from build123d import *

# Parameters (mm, degrees)
ESQUISSE1_W             = 230
ESQUISSE1_H             = 350
BASE_EXTRUSION_DEPTH    = 1.5
ESQUISSE2_R             = 2.5
ENL_V_MAT_EXTRU_1_DEPTH = 1.5
ESQUISSE3_R             = 11.25
ENL_V_MAT_EXTRU_2_DEPTH = 1.5
ESQUISSE4_R             = 6.25
ENL_V_MAT_EXTRU_3_DEPTH = 1.5
ESQUISSE5_W             = 106
ESQUISSE5_H             = 131
ENL_V_MAT_EXTRU_4_DEPTH = 1.5
ESQUISSE6_W             = 37
ESQUISSE6_H             = 46
ENL_V_MAT_EXTRU_5_DEPTH = 1.5


with BuildPart() as part:
    # Esquisse1 → Base-Extrusion (new body)
    with BuildSketch(Plane.XY):
        with Locations((115, 175)):
            Rectangle(ESQUISSE1_W, ESQUISSE1_H)
    extrude(amount=BASE_EXTRUSION_DEPTH)

    # Esquisse2 → Enlèv. mat.-Extru.1 (cut)
    with BuildSketch(Plane.XY.offset(1.5)):
        with Locations((7, 7)):
            Circle(ESQUISSE2_R)
        with Locations((223, 7)):
            Circle(ESQUISSE2_R)
        with Locations((7, 343)):
            Circle(ESQUISSE2_R)
        with Locations((223, 343)):
            Circle(ESQUISSE2_R)
    extrude(amount=-ENL_V_MAT_EXTRU_1_DEPTH, mode=Mode.SUBTRACT)

    # Esquisse3 → Enlèv. mat.-Extru.2 (cut)
    with BuildSketch(Plane.XY.offset(1.5)):
        with Locations((45, 65)):
            Circle(ESQUISSE3_R)
        with Locations((45, 115)):
            Circle(ESQUISSE3_R)
        with Locations((45, 165)):
            Circle(ESQUISSE3_R)
        with Locations((45, 305)):
            Circle(ESQUISSE3_R)
        with BuildLine():
            Line((43.5, 251.14955156), (43.5, 253))
            Line((43.5, 253), (46.5, 253))
            Line((46.5, 253), (46.5, 251.14955156))
            ThreePointArc((46.5, 251.14955156), (45, 228.75), (43.5, 251.14955156))
        make_face()
    extrude(amount=-ENL_V_MAT_EXTRU_2_DEPTH, mode=Mode.SUBTRACT)

    # Esquisse4 → Enlèv. mat.-Extru.3 (cut)
    with BuildSketch(Plane.XY.offset(1.5)):
        with Locations((130, 70)):
            Circle(ESQUISSE4_R)
        with Locations((130, 89)):
            Circle(ESQUISSE4_R)
        with Locations((160, 70)):
            Circle(ESQUISSE4_R)
        with Locations((160, 89)):
            Circle(ESQUISSE4_R)
        with Locations((190, 70)):
            Circle(ESQUISSE4_R)
        with Locations((190, 89)):
            Circle(ESQUISSE4_R)
    extrude(amount=-ENL_V_MAT_EXTRU_3_DEPTH, mode=Mode.SUBTRACT)

    # Esquisse5 → Enlèv. mat.-Extru.4 (cut)
    with BuildSketch(Plane.XY.offset(1.5)):
        with Locations((163, 175.5)):
            Rectangle(ESQUISSE5_W, ESQUISSE5_H)
    extrude(amount=-ENL_V_MAT_EXTRU_4_DEPTH, mode=Mode.SUBTRACT)

    # Esquisse6 → Enlèv. mat.-Extru.5 (cut)
    with BuildSketch(Plane.XY.offset(1.5)):
        with Locations((162.5, 297)):
            Rectangle(ESQUISSE6_W, ESQUISSE6_H)
    extrude(amount=-ENL_V_MAT_EXTRU_5_DEPTH, mode=Mode.SUBTRACT)


solid = part.part
Verification items for the finished model (mm, model axes). Coordinates: 2 decimals unless noted, no trailing zeros. Write each loop counter-clockwise with the first axis right and the second up, starting at its lowest first coordinate (ties: lowest second). Pieces come first, ordered by that corner, then holes. Notation, with made-up numbers: (-6, 52.5) - (42, 52.5) arc R20 cw to (42, 69.5) - close; hole circle Ø11 at (7, 14.25). An arc over 180 degrees is marked (long way). Answer as a JSON object with one key per item and string values.
(1) Cross-section at B-B on x = 190. Record the cut outline in (y, z).
Report:
{"outline": "(0, 0) - (63.75, 0) - (63.75, 1.5) - (0, 1.5) - close; (76.25, 0) - (82.75, 0) - (82.75, 1.5) - (76.25, 1.5) - close; (95.25, 0) - (110, 0) - (110, 1.5) - (95.25, 1.5) - close; (241, 0) - (350, 0) - (350, 1.5) - (241, 1.5) - close"}
(2) Cross-section at D-D on z = 0.25. Give the number of separate pieces and of enclosed holes in the cut face, plus the area to 3 significant figures.
Report:
{"separate pieces": "1", "enclosed holes": "17", "area": "62,100 mm^2"}
(3) Cross-section at C-C on y = 213.5. Record the cut outline in (x, z).
Report:
{"outline": "(0, 0) - (110, 0) - (110, 1.5) - (0, 1.5) - close; (216, 0) - (230, 0) - (230, 1.5) - (216, 1.5) - close"}
(4) Mould release check, pull along Y, two halves, no side actions. Record for faces 1 (the flat face through (88, 177, 1.5)), 2 (the cylindrical face through (43.535, 176.154, 0.76)): pulls with the +Y half, pulls with the -Y half, needs draft (parallel to the pull), parting line crosses it, or undercut.
Report:
{"face 1": "needs draft", "face 2": "undercut"}
(5) Cross-section at A-A on y = 165. Record the cut outline in (x, z).
Report:
{"outline": "(0, 0) - (33.75, 0) - (33.75, 1.5) - (0, 1.5) - close; (56.25, 0) - (110, 0) - (110, 1.5) - (56.25, 1.5) - close; (216, 0) - (230, 0) - (230, 1.5) - (216, 1.5) - close"}
(6) Thickness scan on line 1 along Y through (x, z) = (7, 0.95); line 2 along Y through (x, z) = (45, 0.95); line 3 along Y through (x, z) = (130, 0.8). Record the ranges inside material, lowest first.
Report:
{"line 1": "0 to 4.5, 9.5 to 340.5, 345.5 to 350", "line 2": "0 to 53.75, 76.25 to 103.75, 126.25 to 153.75, 176.25 to 228.75, 253 to 293.75, 316.25 to 350", "line 3": "0 to 63.75, 76.25 to 82.75, 95.25 to 110, 241 to 350"}
